For this review, take the finished solid that the model builds, in its own axes (mm). Face numbers are marked on the shaded views. A direction names the side the tool comes from. Coordinates: 2 decimals unless noted, no trailing zeros. Write each loop counter-clockwise with the first axis right and the second up, starting at its lowest first coordinate (ties: lowest second). Pieces come first, ordered by that corner, then holes.
```python
from build123d import *

# Parameters (mm, degrees)
SKETCH1_R           = 1
SKETCH1_R_2         = 0.625
SKETCH1_R_3         = 2.7
SKETCH1_R_4         = 1.45
SKETCH1_R_5         = 1.112325309
BOSS_EXTRUDE1_DEPTH = 1
SKETCH2_R           = 1.112325309
SKETCH2_R_2         = 1.45
SKETCH2_R_3         = 0.625
SKETCH2_R_4         = 1
BOSS_EXTRUDE2_DEPTH = 9.9
BOSS_EXTRUDE3_DEPTH = 1.55
SKETCH4_R           = 2.2
CUT_EXTRUDE1_DEPTH  = 2.1
SKETCH5_R           = 3.55
SKETCH5_R_2         = 2.7
BOSS_EXTRUDE4_DEPTH = 0.8
SKETCH6_R           = 2.05
BOSS_EXTRUDE5_DEPTH = 2.4
SKETCH7_W           = 5
SKETCH7_H           = 5.2
SKETCH7_R           = 1.1
BOSS_EXTRUDE6_DEPTH = 1.3
CUT_EXTRUDE2_DEPTH  = 1.3
BOSS_EXTRUDE7_DEPTH = 11.7
CUT_EXTRUDE3_DEPTH  = 1.7
SKETCH11_W          = 5.1
SKETCH11_H          = 1.6
BOSS_EXTRUDE8_DEPTH = 3
SKETCH12_W          = 5.1
SKETCH12_H          = 1
BOSS_EXTRUDE9_DEPTH = 2.5
SKETCH13_R          = 1
CUT_EXTRUDE4_DEPTH  = 2.5
FILLET1_R           = 0.3
FILLET2_R           = 0.3


with BuildPart() as part:
    # Sketch1 → Boss-Extrude1 (new body)
    with BuildSketch(Plane.XY):
        with BuildLine():
            Line((-7.55, -18.5), (7.55, -18.5))
            ThreePointArc((7.55, -18.5), (10.095584412, -17.445584412), (11.15, -14.9))
            Line((11.15, -14.9), (11.15, 18.5))
            Line((11.15, 18.5), (-11.15, 18.5))
            Line((-11.15, 18.5), (-11.15, -14.9))
            ThreePointArc((-11.15, -14.9), (-10.095584412, -17.445584412), (-7.55, -18.5))
        make_face()
        with Locations((9.15, -16.5)):
            Circle(SKETCH1_R, mode=Mode.SUBTRACT)
        with Locations((-9.95, -1.55)):
            Circle(SKETCH1_R_2, mode=Mode.SUBTRACT)
        with Locations((9.95, -1.55)):
            Circle(SKETCH1_R_2, mode=Mode.SUBTRACT)
        with Locations((-9.15, -16.5)):
            Circle(SKETCH1_R, mode=Mode.SUBTRACT)
        with Locations((0, -7.2)):
            Circle(SKETCH1_R_3, mode=Mode.SUBTRACT)
        with Locations((9.15, 16.5)):
            Circle(SKETCH1_R, mode=Mode.SUBTRACT)
        with Locations((-9.15, 16.5)):
            Circle(SKETCH1_R, mode=Mode.SUBTRACT)
        with Locations((8.95, 13.456564441)):
            Circle(SKETCH1_R_4, mode=Mode.SUBTRACT)
        with Locations((6.312747808, 15.9)):
            Circle(SKETCH1_R_5, mode=Mode.SUBTRACT)
        with Locations((-6.312747808, 15.9)):
            Circle(SKETCH1_R_5, mode=Mode.SUBTRACT)
        with Locations((-8.95, 13.456564441)):
            Circle(SKETCH1_R_4, mode=Mode.SUBTRACT)
    extrude(amount=BOSS_EXTRUDE1_DEPTH)

    # Sketch2 → Boss-Extrude2 (add)
    with BuildSketch(Plane.XY):
        with BuildLine():
            Line((-11.15, -14.9), (-11.15, 18.5))
            Line((-11.15, 18.5), (11.15, 18.5))
            Line((11.15, 18.5), (11.15, -14.9))
            ThreePointArc((11.15, -14.9), (10.095584412, -17.445584412), (7.55, -18.5))
            Line((7.55, -18.5), (-7.55, -18.5))
            ThreePointArc((-7.55, -18.5), (-10.095584412, -17.445584412), (-11.15, -14.9))
        make_face()
        with Locations((-6.312747808, 15.9)):
            Circle(SKETCH2_R, mode=Mode.SUBTRACT)
        with Locations((-8.95, 13.456564441)):
            Circle(SKETCH2_R_2, mode=Mode.SUBTRACT)
        with Locations((-9.95, -1.55)):
            Circle(SKETCH2_R_3, mode=Mode.SUBTRACT)
        with Locations((-9.15, -16.5)):
            Circle(SKETCH2_R_4, mode=Mode.SUBTRACT)
        with Locations((9.15, -16.5)):
            Circle(SKETCH2_R_4, mode=Mode.SUBTRACT)
        with Locations((9.95, -1.55)):
            Circle(SKETCH2_R_3, mode=Mode.SUBTRACT)
        with Locations((8.95, 13.456564441)):
            Circle(SKETCH2_R_2, mode=Mode.SUBTRACT)
        with Locations((6.312747808, 15.9)):
            Circle(SKETCH2_R, mode=Mode.SUBTRACT)
        with Locations((-9.15, 16.5)):
            Circle(SKETCH2_R_4, mode=Mode.SUBTRACT)
        with Locations((9.15, 16.5)):
            Circle(SKETCH2_R_4, mode=Mode.SUBTRACT)
        with BuildLine():
            Line((-10.15, -14.9), (-10.15, -2.657079491))
            ThreePointArc((-10.15, -2.657079491), (-8.825, -1.55), (-10.15, -0.442920509))
            Line((-10.15, -0.442920509), (-10.15, 11.919521826))
            ThreePointArc((-10.15, 11.919521826), (-7.638269734, 12.013697951), (-7.305911803, 14.505122499))
            ThreePointArc((-7.305911803, 14.505122499), (-4.803101136, 15.091900446), (-5.702782265, 17.5))
            Line((-5.702782265, 17.5), (5.702782265, 17.5))
            ThreePointArc((5.702782265, 17.5), (4.803101136, 15.091900446), (7.305911803, 14.505122499))
            ThreePointArc((7.305911803, 14.505122499), (7.638269734, 12.013697951), (10.15, 11.919521826))
            Line((10.15, 11.919521826), (10.15, -0.442920509))
            ThreePointArc((10.15, -0.442920509), (8.825, -1.55), (10.15, -2.657079491))
            Line((10.15, -2.657079491), (10.15, -14.9))
            ThreePointArc((10.15, -14.9), (10.142584462, -15.096228972), (10.120380146, -15.291338604))
            ThreePointArc((10.120380146, -15.291338604), (8.053984489, -15.403984489), (7.941338604, -17.470380146))
            ThreePointArc((7.941338604, -17.470380146), (7.746228972, -17.492584462), (7.55, -17.5))
            Line((7.55, -17.5), (-7.55, -17.5))
            ThreePointArc((-7.55, -17.5), (-7.746228972, -17.492584462), (-7.941338604, -17.470380146))
            ThreePointArc((-7.941338604, -17.470380146), (-8.053984489, -15.403984489), (-10.120380146, -15.291338604))
            ThreePointArc((-10.120380146, -15.291338604), (-10.142584462, -15.096228972), (-10.15, -14.9))
        make_face(mode=Mode.SUBTRACT)
    extrude(amount=BOSS_EXTRUDE2_DEPTH)

    # Sketch3 → Boss-Extrude3 (add)
    with BuildSketch(Plane.XY.offset(1)):
        with BuildLine():
            Line((5.702782265, 17.5), (4.327174843, 17.5))
            ThreePointArc((4.327174843, 17.5), (4.183564019, 14.496762175), (7.000038147, 13.444367293))
            ThreePointArc((7.000038147, 13.444367293), (7.076340654, 13.996842756), (7.305911803, 14.505122499))
            ThreePointArc((7.305911803, 14.505122499), (4.803101136, 15.091900446), (5.702782265, 17.5))
        make_face()
        with BuildLine():
            Line((-4.327174843, 17.5), (-5.702782265, 17.5))
            ThreePointArc((-5.702782265, 17.5), (-4.803101136, 15.091900446), (-7.305911803, 14.505122499))
            ThreePointArc((-7.305911803, 14.505122499), (-7.076340654, 13.996842756), (-7.000038147, 13.444367293))
            ThreePointArc((-7.000038147, 13.444367293), (-4.183564019, 14.496762175), (-4.327174843, 17.5))
        make_face()
    extrude(amount=BOSS_EXTRUDE3_DEPTH)

    # Sketch4 → Cut-Extrude1 (cut)
    with BuildSketch(Plane(origin=(0, 0, 0), x_dir=(-1, 0, 0), z_dir=(0, 0, -1))):
        with Locations((-6.312747808, 15.9)):
            Circle(SKETCH4_R)
        with Locations((6.312747808, 15.9)):
            Circle(SKETCH4_R)
    extrude(amount=-CUT_EXTRUDE1_DEPTH, mode=Mode.SUBTRACT)

    # Sketch5 → Boss-Extrude4 (add)
    with BuildSketch(Plane(origin=(0, 0, 0), x_dir=(-1, 0, 0), z_dir=(0, 0, -1))):
        with Locations((0, -7.2)):
            Circle(SKETCH5_R)
        with Locations((0, -7.2)):
            Circle(SKETCH5_R_2, mode=Mode.SUBTRACT)
    extrude(amount=BOSS_EXTRUDE4_DEPTH)

    # Sketch6 → Boss-Extrude5 (add)
    with BuildSketch(Plane(origin=(0, 0, 0), x_dir=(-1, 0, 0), z_dir=(0, 0, -1))):
        with Locations((0, 4.45)):
            Circle(SKETCH6_R)
    extrude(amount=BOSS_EXTRUDE5_DEPTH)

    # Sketch7 → Boss-Extrude6 (add)
    with BuildSketch(Plane.XY.offset(9.9)):
        with Locations((0, -21.1)):
            Rectangle(SKETCH7_W, SKETCH7_H)
        with Locations((0, -21.1)):
            Circle(SKETCH7_R, mode=Mode.SUBTRACT)
    extrude(amount=-BOSS_EXTRUDE6_DEPTH)

    # Sketch8 → Cut-Extrude2 (cut)
    with BuildSketch(Plane(origin=(0, 18.5, 0), x_dir=(1, 0, 0), z_dir=(0, 1, 0))):
        with BuildLine():
            Line((3.5, -9.9), (-3.5, -9.9))
            ThreePointArc((-3.5, -9.9), (0, -6.4), (3.5, -9.9))
        make_face()
    extrude(amount=-CUT_EXTRUDE2_DEPTH, mode=Mode.SUBTRACT)

    # Sketch9 → Boss-Extrude7 (add)
    with BuildSketch(Plane(origin=(0, 18.5, 0), x_dir=(1, 0, 0), z_dir=(0, 1, 0))):
        with BuildLine():
            Line((-9.95, -9.9), (-9.95, -9.159245706))
            ThreePointArc((-9.95, -9.159245706), (-10.047335999, -7.629787334), (-9.95, -6.100328962))
            ThreePointArc((-9.95, -6.100328962), (-9.819948204, -5.141444475), (-9.439189189, -4.251840348))
            ThreePointArc((-9.439189189, -4.251840348), (-9.033881062, -3.623934915), (-8.586872248, -3.025))
            ThreePointArc((-8.586872248, -3.025), (-8.2392602, -2.748612181), (-7.806247498, -2.65))
            Line((-7.806247498, -2.65), (7.806247498, -2.65))
            ThreePointArc((7.806247498, -2.65), (8.2392602, -2.748612181), (8.586872248, -3.025))
            ThreePointArc((8.586872248, -3.025), (9.033881062, -3.623934915), (9.439189189, -4.251840348))
            ThreePointArc((9.439189189, -4.251840348), (9.819948204, -5.141444475), (9.95, -6.100328962))
            ThreePointArc((9.95, -6.100328962), (10.047335999, -7.629787334), (9.95, -9.159245706))
            Line((9.95, -9.159245706), (9.95, -9.9))
            Line((9.95, -9.9), (11.15, -9.9))
            Line((11.15, -9.9), (11.15, -8.403337045))
            ThreePointArc((11.15, -8.403337045), (9.935576313, -4.622991063), (7.48348181, -1.5))
            Line((7.48348181, -1.5), (-7.48348181, -1.5))
            ThreePointArc((-7.48348181, -1.5), (-9.935576313, -4.622991063), (-11.15, -8.403337045))
            Line((-11.15, -8.403337045), (-11.15, -9.9))
            Line((-11.15, -9.9), (-9.95, -9.9))
        make_face()
    extrude(amount=BOSS_EXTRUDE7_DEPTH)

    # Sketch10 → Cut-Extrude3 (cut)
    with BuildSketch(Plane.XY.offset(2.65)):
        Polygon((2.55, 24.6), (-2.55, 24.6), (-2.55, 24.95), (-2.9, 24.95), (-2.9, 24.6), (-2.9, 22.4), (2.9, 22.4), (2.9, 24.6), (2.9, 24.95), (2.55, 24.95), align=None)
    extrude(amount=-CUT_EXTRUDE3_DEPTH, mode=Mode.SUBTRACT)

    # Sketch11 → Boss-Extrude8 (add)
    with BuildSketch(Plane(origin=(0, 0, 1.5), x_dir=(-1, 0, 0), z_dir=(0, 0, -1))):
        with Locations((0, 25.4)):
            Rectangle(SKETCH11_W, SKETCH11_H)
    extrude(amount=BOSS_EXTRUDE8_DEPTH)

    # Sketch12 → Boss-Extrude9 (add)
    with BuildSketch(Plane(origin=(0, 26.2, 0), x_dir=(1, 0, 0), z_dir=(0, 1, 0))):
        with Locations((0, 1)):
            Rectangle(SKETCH12_W, SKETCH12_H)
    extrude(amount=-BOSS_EXTRUDE9_DEPTH)

    # Sketch13 → Cut-Extrude4 (cut)
    with BuildSketch(Plane.XY.offset(1)):
        with Locations((0, 4.45)):
            Circle(SKETCH13_R)
    extrude(amount=-CUT_EXTRUDE4_DEPTH, mode=Mode.SUBTRACT)

    # Fillet1
    fillet1_edges = [part.edges().sort_by_distance(p)[0] for p in [
        (2.05, 4.45, -2.4),
    ]]
    fillet(fillet1_edges, radius=FILLET1_R)

    # Fillet2
    fillet2_edges = [part.edges().sort_by_distance(p)[0] for p in [
        (7.48348181, 24.35, 1.5),
        (-7.48348181, 24.35, 1.5),
    ]]
    fillet(fillet2_edges, radius=FILLET2_R)


solid = part.part
```
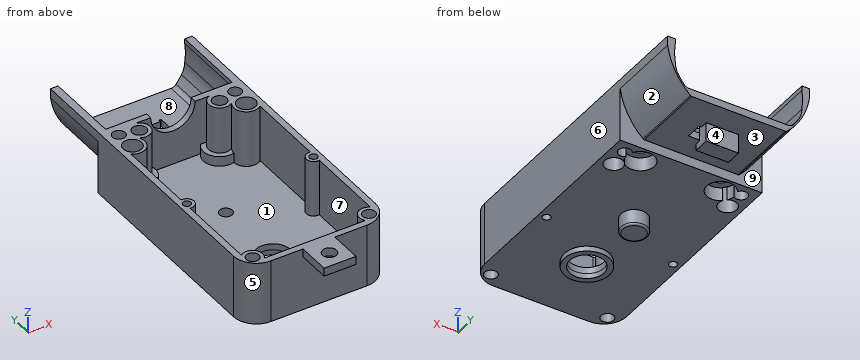
1) The part is to be moulded in two halves that separate along Y. For the marked faces 1, 2, 3 and 4, say which applies: pulls with the +Y half, pulls with the -Y half, needs draft (parallel to the pull), parting line crosses it, or undercut.
2) Consider section C-C (y = -16.5). Give the boundary of the cut face in (x, z), then the cut area to 3 significant figures.
3) Tool access review of the marked faces 5, 6, 7, 8 and 9: name each direction out of +Z, -Z, +X, -X, +Y, -Y from which nothing blocks a thin tool from reaching the whole face with its end or side.
4) Consider section D-D (y = 11). Give the boundary of the cut face in (x, z), then the cut area to 3 significant figures.
5) Consider section A-A (y = -7.2). Give the boundary of the cut face in (x, z).
6) For L1, parallel to Y at x = 0, z = -0.7; L2, parallel to X at y = -17, z = 2; L3, parallel to Y at x = -1, z = 4.25, list the stretches that pass through material, from the lowest coordinate up.
7) Clearance check with flat-ended pins moving along their axes: P1, Ø6, axis at x = 0, y = -7.2, coming from the -Z side; P2, Ø2, axis at x = 0.5, z = 4, coming from the +Y side; P3, Ø2, axis at y = 25, z = 1, coming from the -X side; P4, Ø1.8, axis at x = -9.15, y = 16.5, coming from the +Z side. State where each tip first meets the part, or that it passes through.
8) Consider section B-B (x = 0). Count the separate pieces of the cut face and the enclosed holes in it, then the cut area to 3 significant figures.
Results:
1. face 1: undercut
1. face 2: needs draft
1. face 3: undercut
1. face 4: pulls with the +Y half
2. outline: (-10.77, 0) - (-10.15, 0) - (-10.15, 9.9) - (-10.77, 9.9) - close; (-8.15, 0) - (8.15, 0) - (8.15, 9.9) - (7.6, 9.9) - (7.6, 1) - (-7.6, 1) - (-7.6, 9.9) - (-8.15, 9.9) - close; (10.15, 0) - (10.77, 0) - (10.77, 9.9) - (10.15, 9.9) - close
2. area: 38.5 mm2
3. face 5: +Z, -Z, -X, -Y
3. face 6: +Z, -Z, +X, +Y, -Y
3. face 7: +Z
3. face 8: +Z, +Y
3. face 9: -Z
4. outline: (-11.15, 0) - (11.15, 0) - (11.15, 9.9) - (10.15, 9.9) - (10.15, 1) - (-10.15, 1) - (-10.15, 9.9) - (-11.15, 9.9) - close
4. area: 40.1 mm2
5. outline: (-11.15, 0) - (-3.55, 0) - (-3.55, -0.8) - (-2.7, -0.8) - (-2.7, 1) - (-10.15, 1) - (-10.15, 9.9) - (-11.15, 9.9) - close; (2.7, -0.8) - (3.55, -0.8) - (3.55, 0) - (11.15, 0) - (11.15, 9.9) - (10.15, 9.9) - (10.15, 1) - (2.7, 1) - close
6. L1: y = -10.75 to -9.9, -4.5 to -3.65, 2.4 to 3.45, 5.45 to 6.5, 23.7 to 26.2
6. L2: x = -10.47 to -10.02, -8.28 to -7.68, 7.68 to 8.28, 10.02 to 10.47
6. L3: y = -18.5 to -17.5, 17.5 to 18.5
7. P1: stops at z = -0.8
7. P2: stops at y = 18.5
7. P3: stops at x = -8.01
7. P4: passes through
8. separate pieces: 4
8. enclosed holes: 0
8. area: 72.6 mm2
